CAD build for the part. Positions are in the model's coordinates, mm. A direction names the side the tool comes from. Give positions to 0.01 mm unless a question says otherwise; leave off trailing zeros. Loops run counter-clockwise (first coordinate to the right, second up) from the corner with the lowest first, then second, coordinate; pieces in that order, holes last. Notation, with made-up numbers: M 6.25,-20.5 L 22.25,-20.5 A18 cw 22.25,2.5 Z; hole C -11.5,41.5 d11. An arc over 180 degrees is marked long. Answer as CSV lines item,"result".
```python
from build123d import *

# Parameters (mm, degrees)
EXTRUDE_1_DEPTH          = 50
SKETCH_2_W               = 50
SKETCH_2_H               = 50
EXTRUDE_2_DEPTH          = 2
CUT_EXTRUDE_1_DEPTH      = 46
SKETCH_4_W               = 50
SKETCH_4_H               = 52
EXTRUDE_3_DEPTH          = 2
HOLE_WIZARD_M22_1_D      = 26
HOLE_WIZARD_4_0_4_1_D    = 4
HOLE_WIZARD_M27_1_D      = 30
HOLE_WIZARD_5_0_5_1_D    = 5
FILLET_1_R               = 2
FILLET_2_R               = 3
PATTERN_CIRCULAR_1_COUNT = 4
PATTERN_CIRCULAR_2_COUNT = 4


with BuildPart() as part:
    # 草图1 → 凸台-拉伸1 (new body)
    with BuildSketch(Plane(origin=(46.138674094, 0, 0), x_dir=(0, -1, 0), z_dir=(-1, 0, 0))):
        Polygon((-27, -84.333988555), (-2, -109.333988555), (-2, -84.333988555), align=None)
    extrude(amount=-EXTRUDE_1_DEPTH)

    # 草图2 → 凸台-拉伸2 (add)
    with BuildSketch(Plane.XZ.offset(-2)):
        with Locations((71.138674094, -109.333988555)):
            Rectangle(SKETCH_2_W, SKETCH_2_H)
    extrude(amount=EXTRUDE_2_DEPTH)

    # 草图3 → 切除-拉伸1 (cut)
    with BuildSketch(Plane(origin=(48.138674094, 0, 0), x_dir=(0, -1, 0), z_dir=(-1, 0, 0))):
        Polygon((-2, -84.333988555), (-27, -84.333988555), (-2, -109.333988555), align=None)
    extrude(amount=-CUT_EXTRUDE_1_DEPTH, mode=Mode.SUBTRACT)

    # 草图4 → 凸台-拉伸3 (add)
    with BuildSketch(Plane.XY.offset(-84.333988555)):
        with Locations((71.138674094, 26)):
            Rectangle(SKETCH_4_W, SKETCH_4_H)
    extrude(amount=EXTRUDE_3_DEPTH)

    # M22 间隙孔1 (through all)
    with Locations(Plane(origin=(0, 0, -84.333988555), x_dir=(-1, 0, 0), z_dir=(0, 0, -1))):
        with Locations((-71.138674094, 27)):
            Hole(HOLE_WIZARD_M22_1_D / 2)

    # Ø4.0 (4) 直径孔1 (through all)
    with Locations(Plane(origin=(0, 0, -84.333988555), x_dir=(-1, 0, 0), z_dir=(0, 0, -1))):
        with Locations((-71.138674094, 44.5)):
            hole_wizard_4_0_4_1 = Hole(HOLE_WIZARD_4_0_4_1_D / 2)

    # M27 间隙孔1 (through all)
    with Locations(Plane(origin=(0, 2, 0), x_dir=(1, 0, 0), z_dir=(0, 1, 0))):
        with Locations((71.138674094, 109.333988555)):
            Hole(HOLE_WIZARD_M27_1_D / 2)

    # Ø5.0 (5) 直径孔1 (through all)
    with Locations(Plane(origin=(0, 2, 0), x_dir=(1, 0, 0), z_dir=(0, 1, 0))):
        with Locations((56.138674094, 124.333988555)):
            hole_wizard_5_0_5_1 = Hole(HOLE_WIZARD_5_0_5_1_D / 2)

    # 圆角1
    fillet_1_edges = [part.edges().sort_by_distance(p)[0] for p in [
        (71.138674094, 0, -82.333988555),
    ]]
    fillet(fillet_1_edges, radius=FILLET_1_R)

    # 圆角2
    fillet_2_edges = [part.edges().sort_by_distance(p)[0] for p in [
        (96.138674094, 52, -83.333988555),
        (96.138674094, 1, -134.333988555),
        (46.138674094, 52, -83.333988555),
        (46.138674094, 1, -134.333988555),
    ]]
    fillet(fillet_2_edges, radius=FILLET_2_R)

    # 阵列(圆周)1: Ø5.0 (5) 直径孔1 ×4 about axis
    pattern_circular_1_axis = Axis((71.138674094, 0, -109.333988555), (0, 1, 0))
    for i in range(1, PATTERN_CIRCULAR_1_COUNT):
        add(hole_wizard_5_0_5_1.rotate(pattern_circular_1_axis, i * 360 / PATTERN_CIRCULAR_1_COUNT), mode=Mode.SUBTRACT)

    # 阵列(圆周)2: Ø4.0 (4) 直径孔1 ×4 about axis
    pattern_circular_2_axis = Axis((71.138674094, 27, 0), (0, 0, 1))
    for i in range(1, PATTERN_CIRCULAR_2_COUNT):
        add(hole_wizard_4_0_4_1.rotate(pattern_circular_2_axis, i * 360 / PATTERN_CIRCULAR_2_COUNT), mode=Mode.SUBTRACT)


solid = part.part
```
Q1. Cut at B-B (x = 67.5). Write the cut outline in (y, z).
Solution:
outline,"M 0,-134.33 L 2,-134.33 L 2,-123.89 L 0,-123.89 Z; M 0,-94.78 L 2,-94.78 L 2,-84.33 L 14.52,-84.33 L 14.52,-82.33 L 2,-82.33 A2 ccw 0,-84.33 Z; M 39.48,-84.33 L 52,-84.33 L 52,-82.33 L 39.48,-82.33 Z"
Q2. Pin check, flat tips, straight feed: P1, Ø6, axis at x = 86.14, z = -94.33, coming from the +Y side; P2, Ø12.5, axis at y = 12.5, z = -102.5, coming from the -X side; P3, Ø25, axis at x = 63, y = 26, coming from the -Z side; P4, Ø1.5, axis at x = 73, z = -95.5, coming from the -Y side. Stop position of each tip, or through.
Solution:
P1,"stops at y = 2"
P2,"stops at x = 46.14"
P3,"stops at z = -84.33"
P4,"passes through"
Q3. Wall check: line 1 (Z direction, x = 94.5, y = 48.5); line 2 (Y direction, x = 88.5, z = -91.5). Give the ranges that are in metal, low to high. Write a range as [from, to].
Solution:
line 1,"z = [-84.33, -82.33]"
line 2,"y = [0, 2]"
Q4. Cut at D-D (z = -112). Write the cut outline in (x, y).
Solution:
outline,"M 46.14,0 L 56.38,0 L 56.38,2 L 46.14,2 Z; M 85.9,0 L 96.14,0 L 96.14,2 L 85.9,2 Z"
Q5. Mould opens along Y. For faces 3 (the flat face through (96.139, 12, -94)), 4 (the cylindrical face through (46.994, 51.098, -83.32)), 5 (the cylindrical face through (69.23, 8.9, -83.32)), 6 (the cylindrical face through (90.325, 25.925, -83.32)) say: released by +Y, released by -Y, zero draft, split by the parting line, or undercut.
Solution:
face 3,"zero draft"
face 4,"released by +Y"
face 5,"undercut"
face 6,"undercut"
Q6. Cut at A-A (y = 44.5). Write the cut outline in (x, z).
Solution:
outline,"M 46.14,-84.33 L 69.14,-84.33 L 69.14,-82.33 L 46.14,-82.33 Z; M 73.14,-84.33 L 96.14,-84.33 L 96.14,-82.33 L 73.14,-82.33 Z"
Q7. Cut at C-C (z = -125.5). Write the cut outline in (x, y).
Solution:
outline,"M 46.14,0 L 53.93,0 L 53.93,2 L 46.14,2 Z; M 58.35,0 L 83.93,0 L 83.93,2 L 58.35,2 Z; M 88.35,0 L 96.14,0 L 96.14,2 L 88.35,2 Z"
Q8. Which spindle directions (+Z, -Z, +X, -X, +Y, -Y) get a long thin tool onto all of the face, cutting with end or side? Do faces 1 (the flat face through (46.139, 12, -94)), 2 (the flat face through (60, 2, -98)). Say none if no direction does.
Solution:
face 1,"+Z, -Z, -X, +Y, -Y"
face 2,"-Z, +Y"
